Work out the finished part from the listing and answer in its coordinate system (mm). Face numbers are marked on the shaded views. A direction names the side the tool comes from. Give positions to 0.01 mm unless a question says otherwise; leave off trailing zeros. Order: outer loops, then holes, each group sorted by start corner. A loop starts at its lowest first (then second) coordinate and runs counter-clockwise, first axis right, second up.
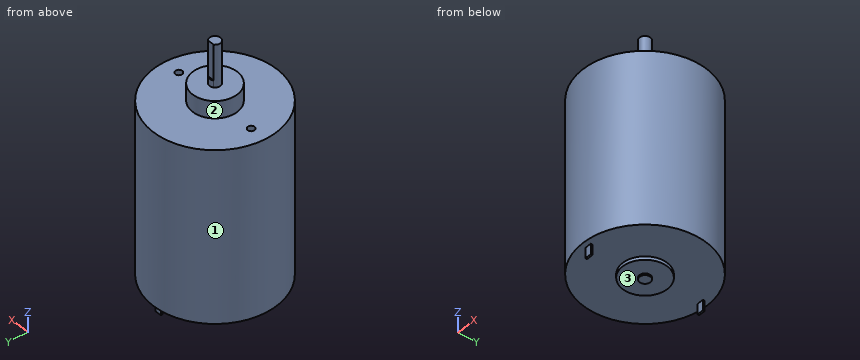
Autodesk Inventor part; units mm, degrees
ref_plane "YZ Plane" through (0, 0, 0) normal (1, 0, 0) x (0, 1, 0)
ref_plane "XZ Plane" through (0, 0, 0) normal (0, 1, 0) x (-1, 0, 0)
ref_plane "XY Plane" through (0, 0, 0) normal (0, 0, 1) x (1, 0, 0)
sketch "Sketch1" plane through (0, 0, 0) normal (0, 0, 1) x (1, 0, 0)
  circle A0 centre (0, 0) radius 18
  circle A1 centre (0, 0) radius 6.5
  arc A2 (-1.0178, 1.215) -> (1.0178, 1.215) centre (0, 0) ccw
  line L0 (-1.585, 0) -> (1.585, 0)
  line L1 (-1.0178, 1.215) -> (1.0178, 1.215)
  circle A3 centre (13, 0) radius 1
  line L2 (0, -18) -> (0, 18) construction
  circle A4 centre (-13, 0) radius 1
  circle A5 centre (0, 0) radius 1.585
  point P0 (1.0178, 1.215)
  point P1 (-1.0178, 1.215)
  dimension "d0" = 36
  dimension "d1" = 13
  dimension "d2" = 3.17
  dimension "d3" = 1.215
  dimension "d4" = 13
  dimension "d5" = 2
  dimension "d6" = 13
  dimension "d7" = 2
  dimension "d36" = 3.17
extrude "Extrusion1" add sketch "Sketch1" along normal blind 17.3 and the other way blind 51.5 contours L1 A2 L0 | L0 A2
extrude "Extrusion2" add sketch "Sketch1" along normal blind 5 and the other way blind 51 contours A1 | A5 L1
extrude "Extrusion3" add sketch "Sketch1" against normal blind 50 contours A0 | A3 | A4
hole "Hole2" at (0, 0, 0) at (13, 0, 0) at (-13, 0, 0) direction (0, 0, -1) diameter 2 depth 8 tip angle 118
thread "Thread1"
thread "Thread2"
extrude "Extrusion4" add sketch "Sketch1" along normal blind 7 and the other way blind 51.5 contours L1 A2 L0 | A5 L1 | L0 A2
sketch "Sketch2" plane through (0, 0, -50) normal (0, 0, -1) x (-1, 0, 0)
  line L0 (-1, 16.45) -> (1, 16.45)
  line L1 (1, 16.45) -> (1, 15.95)
  line L2 (1, 15.95) -> (-1, 15.95)
  line L3 (-1, 15.95) -> (-1, 16.45)
  line L4 (-1, 16.45) -> (1, 15.95) construction
  line L5 (1, 16.45) -> (-1, 15.95) construction
  line L6 (0, 0) -> (0, 18) construction
  circle A0 centre (0, 0) radius 18
  line L7 (0, 0) -> (-18, 0) construction
  line L8 (-1, -16.45) -> (1, -16.45)
  line L9 (1, -16.45) -> (1, -15.95)
  line L10 (1, -15.95) -> (-1, -15.95)
  line L11 (-1, -15.95) -> (-1, -16.45)
  line L12 (-1, -16.45) -> (1, -15.95) construction
  line L13 (1, -16.45) -> (-1, -15.95) construction
  point P0 (0, 16.2)
  point P1 (0, -16.2)
  dimension "d41" = 2
  dimension "d42" = 0.5
extrude "Extrusion5" add sketch "Sketch2" along normal blind 3 contours L0 L1 L2 L3 | L11 L10 L9 L8
properties part number "Motor" material "Stainless Steel"
1. Straight lines are drawn through the part: probe 1 along Z at (x, y) = (-1, -7); probe 2 along Y at (x, z) = (-13, -4.5); probe 3 along Z at (x, y) = (3, 5). For each, find the intervals that lie inside material, in ascending order.
Findings below:
probe 1: z = -50 to 0
probe 2: y = -12.45 to -1, 1 to 12.45
probe 3: z = -51 to 5
2. The part is cut by section B-B (y = 4). Write down the section's boundary in (x, z), then the cut area to 3 significant figures.
Findings below:
outline: (-17.55, -50) - (-5.12, -50) - (-5.12, -51) - (5.12, -51) - (5.12, -50) - (17.55, -50) - (17.55, 0) - (5.12, 0) - (5.12, 5) - (-5.12, 5) - (-5.12, 0) - (-17.55, 0) - close
area: 1,820 mm2
3. The part is cut by section C-C (z = -44). Write down the section's boundary in (x, y).
Findings below:
outline: circle Ø36 at (0, 0)
4. Given P1, Ø2, axis at x = -0.5, z = 13, coming from the +Y side (3 decimals); P2, Ø6, axis at y = -6.5, z = -36.5, coming from the -X side; P3, Ø5, axis at x = 6.5, z = 0, coming from the +Y side; P4, Ø2, axis at x = -14.5, y = -12.5, coming from the +Z side, each flat-ended and moving along its own axis, determine where each tip first touches the part or whether it passes through.
Findings below:
P1: stops at y = 1.215
P2: stops at x = -17.66
P3: stops at y = 17.55
P4: passes through
5. Which of the six approach directions +Z, -Z, +X, -X, +Y, -Y give full straight-line access (tool end or side, diameter ignored) to the marked faces 1, 2 and 3?
Findings below:
face 1: +Z, -Z
face 2: +Z
face 3: -Z
6. The part is cut by section D-D (x = 4.5). Write down the section's boundary in (y, z).
Findings below:
outline: (-17.43, -50) - (-4.69, -50) - (-4.69, -51) - (4.69, -51) - (4.69, -50) - (17.43, -50) - (17.43, 0) - (4.69, 0) - (4.69, 5) - (-4.69, 5) - (-4.69, 0) - (-17.43, 0) - close
